Autodesk Fusion 360 part; units mm, degrees
sketch "Sketch1" plane through (0, 0, 0) normal (0, 0, 1) x (1, 0, 0)
  circle A0 centre (0, 0) radius 6.45
  circle A1 centre (0, 0) radius 6.35
  circle A2 centre (0, 0) radius 8.95
  line L0 (0, 0) -> (0, 5)
  line L1 (0, 5) -> (7.4231, 5)
  line L2 (7.4231, 5) -> (77.4231, 5)
  line L3 (77.4231, 5) -> (77.4231, -5)
  line L4 (77.4231, -5) -> (7.4231, -5)
  line L5 (7.4231, -5) -> (7.4231, 5)
  dimension "d1" = 12.9
  dimension "d2" = 12.7
  dimension "d3" = 17.9
  dimension "d4" = 5
  dimension "d5" = 70
  dimension "d6" = 10
extrude "Extrude2" add sketch "Sketch1" along normal blind 10 and the other way blind 10 contours A2 L5 | A2 L5
extrude "Extrude3" add sketch "Sketch1" along normal blind 5 and the other way blind 5 contours A2 L2 L3 L4
fillet "Fillet1" radius 0.5 4 edges at (42.4231, -5, 5) (42.4231, -5, -5) (42.4231, 5, -5) (42.4231, 5, 5) 1 faces at (77.4231, 1.6667, -1.6667)
The model under review builds one solid part; all positions refer to its coordinate system, in mm. A direction names the side the tool comes from. Round coordinates to 2 decimals unless told otherwise and drop trailing zeros. Loops run counter-clockwise (first coordinate to the right, second up) from the corner with the lowest first, then second, coordinate; pieces in that order, holes last. Notation, with made-up numbers: (27, 21.5) - (82, 21.5) arc R17 ccw to (82, 35.5) - close; hole circle Ø3 at (36.5, 74.25). An arc over 180 degrees is marked (long way). Write each question's results on one line, items separated by ' | '. Start each with the question number.
Q1. Take a section at D-D on x = 23. Give the boundary of the cut face in (y, z), plus the area to 3 significant figures.
Q2. Take a section at A-A on x = 0. Give the boundary of the cut face in (y, z).
Q3. Tool access review of faces 1 (the flat face through (77.423, 0, 0)), 2 (the flat face through (43, -5, 0)), 3 (the flat face through (42, 5, 0)): name each direction out of +Z, -Z, +X, -X, +Y, -Y from which nothing blocks a thin tool from reaching the whole face with its end or side.
Q4. Draft analysis for pull direction Y (two halves, no side actions). For faces 4 (the cylindrical face through (-1.398, 6.297, -0.14)), 5 (the flat face through (3, -6, 10)), 6 (the cylindrical face through (-8.94, -0.39, -0.14)), state which applies: pulls with the +Y half, pulls with the -Y half, needs draft (parallel to the pull), parting line crosses it, or undercut.
Q5. Wall thickness on line 1 along X through (y, z) = (0, 3.5); line 2 along Y through (x, z) = (0, -3.25); line 3 along Z through (x, y) = (65, -4): over which ranges is each line inside the solid? List them lowest first. Write a range as [from, to].
Q6. Take a section at C-C on y = 0. Give the boundary of the cut face in (x, z), plus the area to 3 significant figures.
Q7. Take a section at B-B on z = 1.5. Give the boundary of the cut face in (x, y).
Q8. Insertion check: P1, Ø1.5, axis at y = -1.5, z = 7, coming from the +X side; P2, Ø7, axis at x = 38, z = 0.5, coming from the +Y side; P3, Ø7, axis at x = 36, z = -2, coming from the -Y side. Each pin has a flat end and moves straight along its axis. Give the tip position at first contact, or say it passes through.
Data:
1) outline: (-5, -4.5) arc R0.5 ccw to (-4.5, -5) - (4.5, -5) arc R0.5 ccw to (5, -4.5) - (5, 4.5) arc R0.5 ccw to (4.5, 5) - (-4.5, 5) arc R0.5 ccw to (-5, 4.5) - close | area: 99.8 mm²
2) outline: (-8.95, -10) - (-6.45, -10) - (-6.45, 10) - (-8.95, 10) - close; (6.45, -10) - (8.95, -10) - (8.95, 10) - (6.45, 10) - close
3) face 1: +Z, -Z, +X, +Y, -Y | face 2: +Z, -Z, +X, -Y | face 3: +Z, -Z, +X, +Y
4) face 4: undercut | face 5: needs draft | face 6: parting line crosses it
5) line 1: x = [-8.95, -6.45], [6.45, 77.42] | line 2: y = [-8.95, -6.45], [6.45, 8.95] | line 3: z = [-5, 5]
6) outline: (-8.95, -10) - (-6.45, -10) - (-6.45, 10) - (-8.95, 10) - close; (6.45, -10) - (8.95, -10) - (8.95, -5) - (76.92, -5) arc R0.5 ccw to (77.42, -4.5) - (77.42, 4.5) arc R0.5 ccw to (76.92, 5) - (8.95, 5) - (8.95, 10) - (6.45, 10) - close | area: 785 mm²
7) outline: (7.42, -5) - (76.92, -5) arc R0.5 ccw to (77.42, -4.5) - (77.42, 4.5) arc R0.5 ccw to (76.92, 5) - (7.42, 5) arc R8.95 ccw (long way) to start; hole circle Ø12.9 at (0, 0)
8) P1: stops at x = 8.92 | P2: stops at y = 5 | P3: stops at y = -5
